Geometry check sheet. Reference: the model listing, model coordinates, mm. A direction names the side the tool comes from. Give positions to 0.01 mm unless a question says otherwise; leave off trailing zeros. Order: outer loops, then holes, each group sorted by start corner. A loop starts at its lowest first (then second) coordinate and runs counter-clockwise, first axis right, second up. Notation, with made-up numbers: M 75,37 L 113,37 A13 ccw 113,60 Z; hole C -28,61.5 d3. An arc over 180 degrees is marked long. Answer as a JSON object with one key per item and string values. Group by question number.
from build123d import *

# Parameters (mm, degrees)
EXTRUDE1_DEPTH              = 6.35
SKETCH2_W                   = 17.047492734
SKETCH2_H                   = 1.5875
EXTRUDE2_DEPTH              = 7.35
SKETCH4_R                   = 3.175
EXTRUDE4_DEPTH              = 7.35
FILLET2_R                   = 4.318
F_32_0_116_DIAMETER_HOLE1_D = 2.9464
EXTRUDE8_DEPTH              = 28.6766
FILLET1_R                   = 2.54


with BuildPart() as part:
    # Sketch1 → Extrude1 (new body)
    with BuildSketch(Plane.XY):
        Polygon((-21.492492734, 7.62), (-6.252492734, 7.62), (1.367507266, 7.62), (1.367507266, 0), (1.367507266, -7.62), (-6.252492734, -7.62), (-21.492492734, -7.62), align=None)
    extrude(amount=EXTRUDE1_DEPTH)

    # Sketch2 → Extrude2 (cut, through all)
    with BuildSketch(Plane.XY.offset(6.35)):
        with Locations((-12.968746367, 0)):
            Rectangle(SKETCH2_W, SKETCH2_H)
    extrude(amount=-EXTRUDE2_DEPTH, mode=Mode.SUBTRACT)

    # Sketch4 → Extrude4 (cut, through all)
    with BuildSketch(Plane.XY.offset(6.35)):
        with Locations((-8.89, 0)):
            Circle(SKETCH4_R)
    extrude(amount=-EXTRUDE4_DEPTH, mode=Mode.SUBTRACT)

    # Fillet2
    fillet2_edges = [part.edges().sort_by_distance(p)[0] for p in [
        (1.367507266, 7.62, 3.175),
        (1.367507266, -7.62, 3.175),
    ]]
    fillet(fillet2_edges, radius=FILLET2_R)

    # #32 (0.116) Diameter Hole1 (through all)
    with Locations(Plane(origin=(-18.444492734, -7.62, 3.175), x_dir=(0, 0, -1), z_dir=(0, -1, 0))):
        with Locations((0, 0)):
            Hole(F_32_0_116_DIAMETER_HOLE1_D / 2)

    # Sketch21 → Extrude8 (add)
    with BuildSketch(Plane(origin=(0, 7.62, 0), x_dir=(1, 0, 0), z_dir=(0, 1, 0))):
        Polygon((-8.89, 0), (-4.826, 0), (-4.826, -6.35), (-12.954, -6.35), (-12.954, 0), align=None)
    extrude8 = extrude(amount=EXTRUDE8_DEPTH)

    # Sketch27 → #50 (0.07) Diameter Hole1 (revolve, cut)
    with BuildSketch(Plane(origin=(-8.89, 31.75, 0), x_dir=(0, 1, 0), z_dir=(1, 0, 0))):
        Polygon((0, 0), (0, 6.88416509), (0.889, 6.35), (0.889, 0), align=None)
    f_50_0_07_diameter_hole1 = revolve(axis=Axis((-8.89, 31.75, -6.35), (0, 0, 1)), mode=Mode.SUBTRACT)

    # Mirror2: Extrude8, #50 (0.07) Diameter Hole1 across plane
    add(extrude8.mirror(Plane.ZX))
    add(f_50_0_07_diameter_hole1.mirror(Plane.ZX), mode=Mode.SUBTRACT)

    # Fillet1
    fillet1_edges = [part.edges().sort_by_distance(p)[0] for p in [
        (-12.954, 7.62, 3.175),
        (-4.826, 7.62, 3.175),
        (-12.954, 36.2966, 3.175),
        (-4.826, 36.2966, 3.175),
        (-12.954, -36.2966, 3.175),
        (-12.954, -7.62, 3.175),
        (-4.826, -7.62, 3.175),
        (-4.826, -36.2966, 3.175),
    ]]
    fillet(fillet1_edges, radius=FILLET1_R)


solid = part.part
1. Thickness scan on line 1 along Y through (x, z) = (-8.89, 1.5) (3 decimals); line 2 along X through (y, z) = (31.75, 4.75); line 3 along X through (y, z) = (-23.5, 1.75). Record the ranges inside material, lowest first. Write a range as [from, to].
2. Cross-section at C-C (y = 2). State how many separate pieces and enclosed holes the cut face has, and give its area (3 significant figures).
3. Depth check by flat-ended pin: pin 1 (1.3 mm diameter, centred on y = 0, z = 3, fed in from -X) (3 decimals); pin 2 (1.5 mm diameter, centred on x = -5, z = 2, fed in from -Y); pin 3 (1.9 mm diameter, centred on y = 26, z = 4, fed in from -X); pin 4 (1.5 mm diameter, centred on x = -3, y = -14.5, fed in from -Z). Enter the tip coordinate at first touch or a pass-through.
4. Cross-section at B-B (x = -8.89). Record the cut outline in (y, z) (3 decimals).
5. Cross-section at A-A (y = 31.75). Record the cut outline in (x, z), and give its area (3 significant figures).
6. Access from +Z, -Z, +X, -X, +Y, -Y to the whole of each face (thin tool, end or side, straight path). Record for faces 4 (the flat face through (-4.826, -22, 3)), 5 (the flat face through (-5, 0.794, 3)), 6 (the flat face through (-12.954, 22, 3)).
7. Release check for a two-part mould opening along Y. For faces 1 (the flat face through (-9, -36.297, 3)), 2 (the flat face through (-9, 36.297, 3)), 3 (the flat face through (-16.8, -0.794, 3.2)) record: released by +Y, released by -Y, zero draft, split by the parting line, or undercut.
Report:
{
 "1": {"line 1": "y = [-36.297, -32.639], [-30.861, -3.175], [3.175, 30.861], [32.639, 36.297]", "line 2": "x = [-12.95, -9.78], [-8, -4.83]", "line 3": "x = [-12.95, -4.83]"},
 "2": {"separate pieces": "2", "enclosed holes": "1", "area": "107 mm2"},
 "3": {"pin 1": "stops at x = -4.445", "pin 2": "stops at y = -35.72", "pin 3": "stops at x = -12.95", "pin 4": "passes through"},
 "4": {"outline": "M -36.297,0 L -32.639,0 L -32.639,6.35 L -36.297,6.35 Z; M -30.861,0 L -3.175,0 L -3.175,6.35 L -30.861,6.35 Z; M 3.175,0 L 30.861,0 L 30.861,6.35 L 3.175,6.35 Z; M 32.639,0 L 36.297,0 L 36.297,6.35 L 32.639,6.35 Z"},
 "5": {"outline": "M -12.95,0 L -9.78,0 L -9.78,6.35 L -12.95,6.35 Z; M -8,0 L -4.83,0 L -4.83,6.35 L -8,6.35 Z", "area": "40.3 mm2"},
 "6": {"face 4": "+Z, -Z, +X, -Y", "face 5": "+Z, -Z, -X", "face 6": "+Z, -Z, -X, +Y"},
 "7": {"face 1": "released by -Y", "face 2": "released by +Y", "face 3": "undercut"}
}
